Can you work these out from the drawing? Everything is in mm from the part's minimum corner. A direction names the side the tool comes from. Round coordinates to 2 decimals unless told otherwise and drop trailing zeros. Write each loop counter-clockwise with the first axis right and the second up, starting at its lowest first coordinate (ties: lowest second). Pieces come first, ordered by that corner, then holes. Notation, with made-up numbers: (79.25, 2.25) -> (115.25, 2.25) arc R13 cw to (115.25, 8.25) -> close; hole circle Ø3 at (-35.5, 60.5). An arc over 180 degrees is marked (long way). Write item = value, one per line. Start each with the question number.
1) For the marked faces 5, 6, 7, 8 and 9, which set-ups out of +Z, -Z, +X, -X, +Y, -Y let a thin tool reach every point of the face, with its end or its side?
2) If I drill on line 1 (Z direction, x = 284.5, y = 63.5); line 2 (X direction, y = 87.5, z = 56.5); line 3 (Y direction, x = 208, z = 10.5) (1 decimal), over which ranges is the centre line in solid material (lowest first)?
3) Imagine slicing it at A-A, the plane x = 202.5. Please give me the cut outline in (y, z) (1 decimal).
4) Imagine slicing it at D-D, the plane z = 85.5. Please give me the cut outline in (x, y).
5) I'm going to push flat-ended pins straight in: pin 1 (12.5 mm diameter, centred on x = 285, y = 117.5, fed in from +Z); pin 2 (1.5 mm diameter, centred on x = 115, y = 50.5, fed in from +Z). Where does each tip first touch, or does it pass through?
6) Imagine slicing it at B-B, the plane z = 48. Please give me the cut outline in (x, y), then the cut area to 3 significant figures.
7) Thinking about a two-plate mould opening in X: for the marked faces 1, 2, 3 and 4, which applies, +X half, -X half, draft (parallel to the pull), parting line (faces both ways), or undercut?
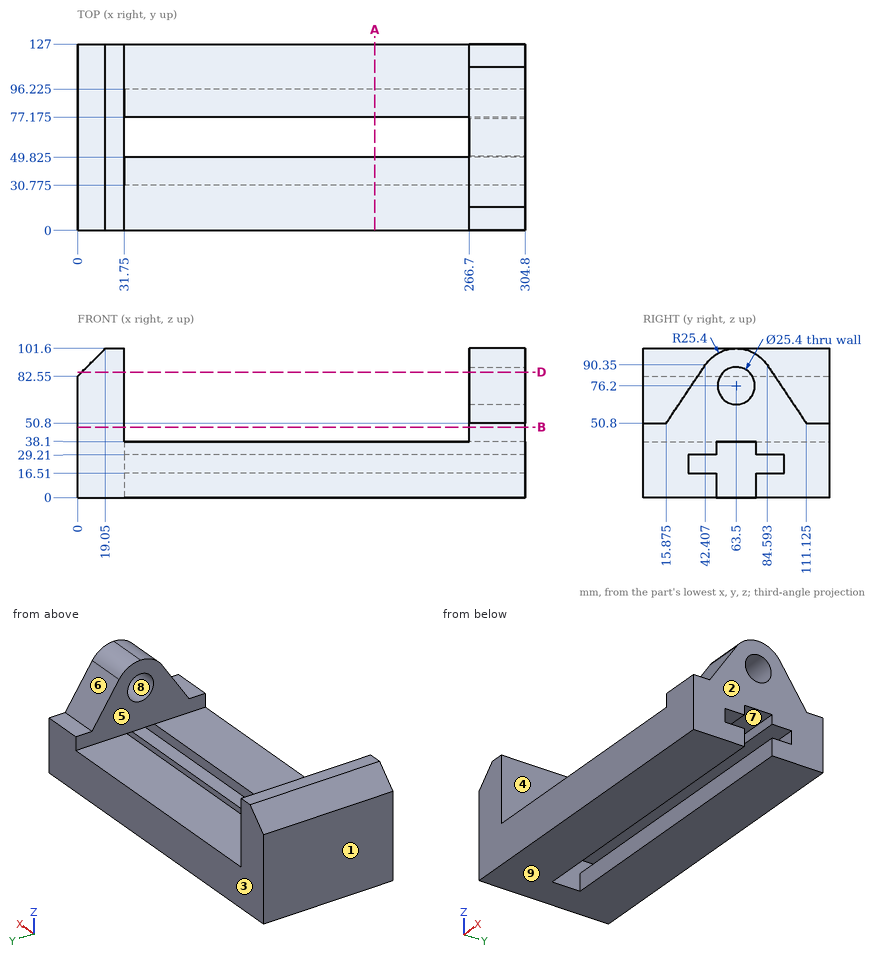
Reported:
q1.face_5 = +Z, +Y, -Y
q1.face_6 = +Z, +X, +Y
q1.face_7 = -Z, +X
q1.face_8 = +X
q1.face_9 = -Z, +X, -X, +Y, -Y
q2.line_1 = 38.1 to 63.5, 88.9 to 101.6
q2.line_2 = 0 to 31.75, 266.7 to 304.8
q2.line_3 = 0 to 49.8, 77.2 to 127
q3.outline = (0, 0) -> (49.8, 0) -> (49.8, 16.5) -> (30.8, 16.5) -> (30.8, 29.2) -> (49.8, 29.2) -> (49.8, 38.1) -> (0, 38.1) -> close; (77.2, 0) -> (127, 0) -> (127, 38.1) -> (77.2, 38.1) -> (77.2, 29.2) -> (96.2, 29.2) -> (96.2, 16.5) -> (77.2, 16.5) -> close
q4.outline = (2.95, 0) -> (31.75, 0) -> (31.75, 127) -> (2.95, 127) -> close; (266.7, 39.15) -> (304.8, 39.15) -> (304.8, 54.85) -> (266.7, 54.85) -> close; (266.7, 72.15) -> (304.8, 72.15) -> (304.8, 87.85) -> (266.7, 87.85) -> close
q5.pin_1 = 50.8
q5.pin_2 = 38.1
q6.outline = (0, 0) -> (31.75, 0) -> (31.75, 127) -> (0, 127) -> close; (266.7, 0) -> (304.8, 0) -> (304.8, 127) -> (266.7, 127) -> close
q6.area = 8,870 mm²
q7.face_1 = -X half
q7.face_2 = +X half
q7.face_3 = draft
q7.face_4 = undercut
